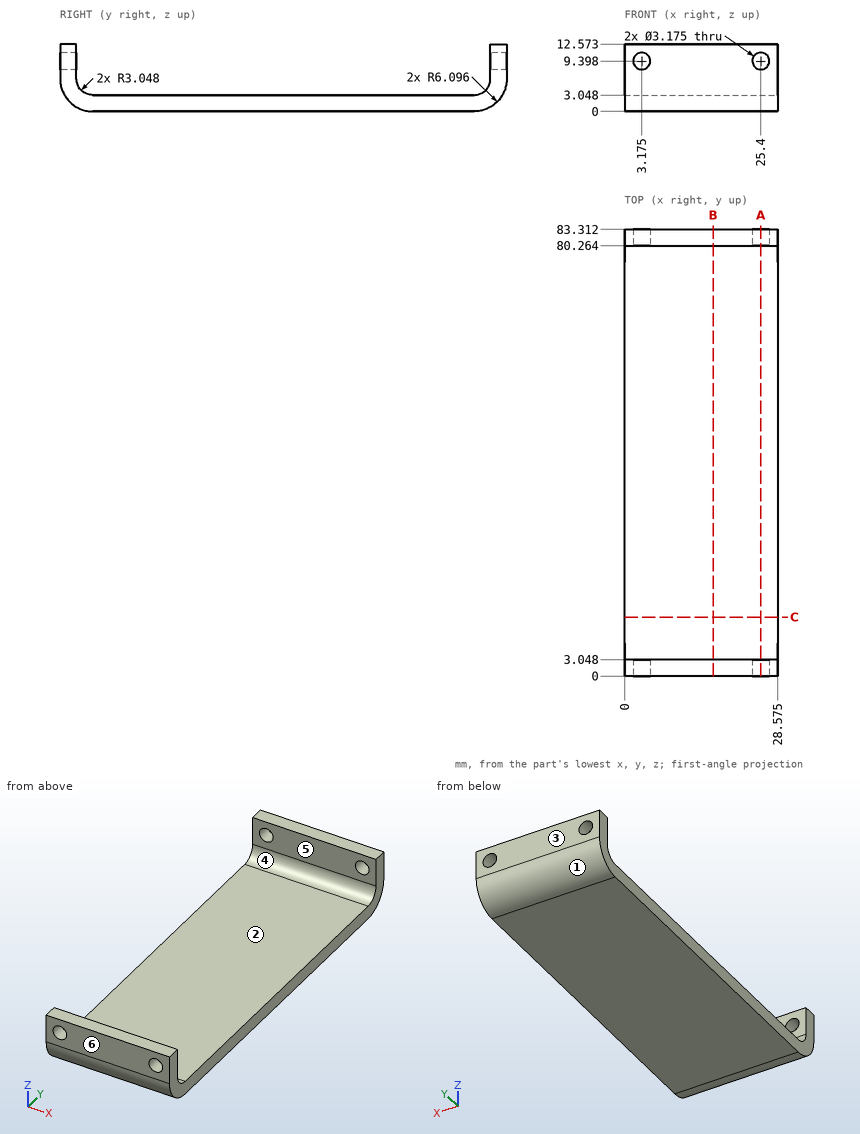
Can you work these out from the drawing? Everything is in mm from the part's minimum corner. A direction names the side the tool comes from. Round coordinates to 2 decimals unless told otherwise and drop trailing zeros. Write each loop counter-clockwise with the first axis right and the second up, starting at its lowest first coordinate (ties: lowest second). Pieces come first, ordered by that corner, then holes. Notation, with made-up numbers: (89.25, 61) - (105.25, 61) arc R19 ccw to (105.25, 73) - close; hole circle Ø10 at (-6, -16.75). An arc over 180 degrees is marked (long way). Use a Markdown table: item, result.
Q1. I want a section at C-C (y = 11). List the corners of the cut face in (x, z) for me (3 decimals), plus the area to 3 significant figures.
Output values:
| item | result |
|---|---|
| outline | (0, 0) - (28.575, 0) - (28.575, 3.048) - (0, 3.048) - close |
| area | 87.1 mm2 |
Q2. Thinking about a two-plate mould opening in Y: for the marked faces 3, 4, 5 and 6, which applies, released by +Y, released by -Y, zero draft, split by the parting line, or undercut?
Output values:
| item | result |
|---|---|
| face 3 | released by +Y |
| face 4 | undercut |
| face 5 | undercut |
| face 6 | released by -Y |
Q3. I want a section at B-B (x = 16.5). List the corners of the cut face in (y, z) for me.
Output values:
| item | result |
|---|---|
| outline | (0, 6.1) arc R6.1 ccw to (6.1, 0) - (77.22, 0) arc R6.1 ccw to (83.31, 6.1) - (83.31, 12.57) - (80.26, 12.57) - (80.26, 6.1) arc R3.05 cw to (77.22, 3.05) - (6.1, 3.05) arc R3.05 cw to (3.05, 6.1) - (3.05, 12.57) - (0, 12.57) - close |
Q4. For pin 1 (5 mm diameter, centred on x = 13, y = 65, fed in from +Z); pin 2 (3 mm diameter, centred on x = 21, z = 2, fed in from -Y), each with a flat end and sliding along its axis, tell me the tip position at first contact or that it passes through.
Output values:
| item | result |
|---|---|
| pin 1 | z = 3.05 |
| pin 2 | y = 0.58 |
Q5. For the marked faces 1 and 2, which set-ups out of +Z, -Z, +X, -X, +Y, -Y let a thin tool reach every point of the face, with its end or its side?
Output values:
| item | result |
|---|---|
| face 1 | -Z, +X, -X, +Y |
| face 2 | +Z, +X, -X |
Q6. Please list where these lines run through material, in increasing order: L1, parallel to Y at x = 10.5, z = 12; L2, parallel to Z at x = 10.5, y = 43; L3, parallel to Y at x = 1.25, z = 4.25.
Output values:
| item | result |
|---|---|
| L1 | 0 to 3.05, 80.26 to 83.31 |
| L2 | 0 to 3.05 |
| L3 | 0.29 to 3.67, 79.64 to 83.03 |
Q7. I want a section at A-A (x = 25.4). List the corners of the cut face in (y, z) for me, plus the area to 3 significant figures.
Output values:
| item | result |
|---|---|
| outline | (0, 6.1) arc R6.1 ccw to (6.1, 0) - (77.22, 0) arc R6.1 ccw to (83.31, 6.1) - (83.31, 7.81) - (80.26, 7.81) - (80.26, 6.1) arc R3.05 cw to (77.22, 3.05) - (6.1, 3.05) arc R3.05 cw to (3.05, 6.1) - (3.05, 7.81) - (0, 7.81) - close; (0, 10.99) - (3.05, 10.99) - (3.05, 12.57) - (0, 12.57) - close; (80.26, 10.99) - (83.31, 10.99) - (83.31, 12.57) - (80.26, 12.57) - close |
| area | 281 mm2 |
